Model file for the job. Use its own axes, mm. Face numbers are marked on the shaded views. A direction names the side the tool comes from. Give positions to 0.01 mm unless a question says otherwise; leave off trailing zeros. Order: outer loops, then holes, each group sorted by start corner. A loop starts at its lowest first (then second) coordinate and runs counter-clockwise, first axis right, second up. Notation, with made-up numbers: (47, 57) -> (106, 57) arc R20 ccw to (106, 88) -> close; hole circle Ø4 at (32.25, 1.5). An arc over 180 degrees is marked (long way). Use CSV: the item, a comma, the result in double quotes. Start each with the question number.
1. Pull direction Y, two halves, no side cores. Call the marked faces 1, 2 and 3: released by +Y, released by -Y, zero draft, split by the parting line, or undercut.
2. Cut at C-C on z = 22.25. List the corners of the cut face in (x, y).
3. Wall check: line 1 (Y direction, x = 0, z = 6.8); line 2 (Y direction, x = 0, z = 16.1); line 3 (Y direction, x = -1, z = 8.5). Give the ranges that are in metal, low to high. Write a range as from..to.
4. 3-axis set-ups, long thin cutter, end or side, ignore diameter. For the marked faces 4, 5 and 6: which of +Z, -Z, +X, -X, +Y, -Y reach the whole face in a straight line?
5. Cut at B-B on y = 75. List the corners of the cut face in (x, z).
6. Cut at D-D on x = 56. List the corners of the cut face in (y, z), then the cut area to 3 significant figures.
7. Drop flat-ended pins along their axis: pin 1 (8 mm diameter, centred on x = -50, z = 14.5, fed in from -Y); pin 2 (18 mm diameter, centred on x = 0, y = 110, fed in from -Z); pin 3 (15 mm diameter, centred on x = 51, z = 20.5, fed in from +Y); pin 4 (1 mm diameter, centred on y = 80.5, z = 9.5, fed in from +X). Give the stop position or say it passes through.
8. Cut at A-A on x = 0. List the corners of the cut face in (y, z).
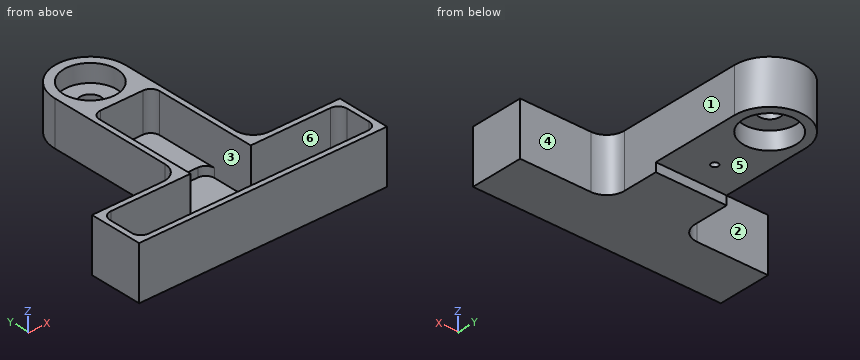
```python
from build123d import *

# Parameters (mm, degrees)
F1_DEPTH  = 30
F2_W      = 40
F2_H      = 70
F3_DEPTH  = 5
F5_DEPTH  = 27
F6_W      = 34
F6_H      = 35
F7_DEPTH  = 22
F8_R      = 15
F9_DEPTH  = 10
F10_R     = 6
F11_DEPTH = 30.001
F12_R     = 10
F13_R     = 5
F14_R     = 15
F15_DEPTH = 10
F16_R     = 2
F17_DEPTH = 8.001


with BuildPart() as f1:
    # F0 (on Top) → F1 (new body)
    with BuildSketch(Plane.XY):
        with BuildLine():
            Line((20, 30), (20, 110))
            ThreePointArc((20, 110), (0, 130), (-20, 110))
            Line((-20, 110), (-20, 30))
            Line((-20, 30), (-70, 30))
            Line((-70, 30), (-70, 0))
            Line((-70, 0), (70, 0))
            Line((70, 0), (70, 30))
            Line((70, 30), (20, 30))
        make_face()
    extrude(amount=F1_DEPTH)

    # F2 (on face) → F3 (cut)
    with BuildSketch(Plane.XY):
        with Locations((0, 95)):
            Rectangle(F2_W, F2_H)
    extrude(amount=F3_DEPTH, mode=Mode.SUBTRACT)

    # F4 (on face) → F5 (cut)
    with BuildSketch(Plane.XY.offset(30)):
        Polygon((-17, 55), (-17, 27), (-67, 27), (-67, 3), (67, 3), (67, 27), (17, 27), (17, 55), align=None)
    extrude(amount=-F5_DEPTH, mode=Mode.SUBTRACT)

    # F6 (on face) → F7 (cut)
    with BuildSketch(Plane.XY.offset(30)):
        with Locations((0, 72.5)):
            Rectangle(F6_W, F6_H)
    extrude(amount=-F7_DEPTH, mode=Mode.SUBTRACT)

    # F8 (on face) → F9 (cut)
    with BuildSketch(Plane.XY.offset(30)):
        with Locations((0, 110)):
            Circle(F8_R)
    extrude(amount=-F9_DEPTH, mode=Mode.SUBTRACT)

    # F10 (on face) → F11 (cut, through all)
    with BuildSketch(Plane.XY.offset(30)):
        with Locations((0, 110)):
            Circle(F10_R)
    extrude(amount=-F11_DEPTH, mode=Mode.SUBTRACT)

    # F12
    f12_edges = [f1.edges().sort_by_distance(p)[0] for p in [
        (20, 30, 15),
        (-20, 30, 15),
    ]]
    fillet(f12_edges, radius=F12_R)

    # F13
    f13_edges = [f1.edges().sort_by_distance(p)[0] for p in [
        (-17, 90, 19),
        (-67, 27, 16.5),
        (17, 90, 19),
        (67, 27, 16.5),
        (-67, 3, 16.5),
        (67, 3, 16.5),
        (-17, 55, 5.5),
        (17, 55, 5.5),
    ]]
    fillet(f13_edges, radius=F13_R)

    # F14 (on face) → F15 (cut)
    with BuildSketch(Plane(origin=(0, 0, 5), x_dir=(1, 0, 0), z_dir=(0, 0, -1))):
        with Locations((0, -110)):
            Circle(F14_R)
    extrude(amount=-F15_DEPTH, mode=Mode.SUBTRACT)

    # F16 (on face) → F17 (cut, through all)
    with BuildSketch(Plane.XY.offset(8)):
        with Locations((0, 75)):
            Circle(F16_R)
    extrude(amount=-F17_DEPTH, mode=Mode.SUBTRACT)


solid = f1.part
```
Verdict:
1,face 1,"zero draft"
1,face 2,"released by +Y"
1,face 3,"undercut"
2,outline,"(-70, 0) -> (70, 0) -> (70, 30) -> (30, 30) arc R10 cw to (20, 40) -> (20, 110) arc R20 ccw to (-20, 110) -> (-20, 40) arc R10 cw to (-30, 30) -> (-70, 30) -> close; hole (-67, 8) arc R5 ccw to (-62, 3) -> (62, 3) arc R5 ccw to (67, 8) -> (67, 22) arc R5 ccw to (62, 27) -> (17, 27) -> (17, 85) arc R5 ccw to (12, 90) -> (-12, 90) arc R5 ccw to (-17, 85) -> (-17, 27) -> (-62, 27) arc R5 ccw to (-67, 22) -> close; hole circle Ø30 at (0, 110)"
3,line 1,"0..3, 55..73, 77..95, 125..130"
3,line 2,"0..3, 90..104, 116..130"
3,line 3,"0..3, 90..95.03, 124.97..129.97"
4,face 4,"+Z, -Z, +X, +Y"
4,face 5,"-Z, +X, -X, +Y"
4,face 6,"+Z"
5,outline,"(-20, 5) -> (-2, 5) -> (-2, 8) -> (-17, 8) -> (-17, 30) -> (-20, 30) -> close; (2, 5) -> (20, 5) -> (20, 30) -> (17, 30) -> (17, 8) -> (2, 8) -> close"
6,outline,"(0, 0) -> (30, 0) -> (30, 30) -> (27, 30) -> (27, 3) -> (3, 3) -> (3, 30) -> (0, 30) -> close"
6,area,"252 mm^2"
7,pin 1,"y = 0"
7,pin 2,"z = 15"
7,pin 3,"y = 30"
7,pin 4,"x = 20"
8,outline,"(0, 0) -> (60, 0) -> (60, 5) -> (73, 5) -> (73, 8) -> (55, 8) -> (55, 3) -> (3, 3) -> (3, 30) -> (0, 30) -> close; (77, 5) -> (95, 5) -> (95, 15) -> (104, 15) -> (104, 20) -> (95, 20) -> (95, 30) -> (90, 30) -> (90, 8) -> (77, 8) -> close; (116, 15) -> (125, 15) -> (125, 5) -> (130, 5) -> (130, 30) -> (125, 30) -> (125, 20) -> (116, 20) -> close"
